Design review of the part built by this model. Coordinates are the model's own, in mm. A direction names the side the tool comes from. Give positions to 0.01 mm unless a question says otherwise; leave off trailing zeros. Loops run counter-clockwise (first coordinate to the right, second up) from the corner with the lowest first, then second, coordinate; pieces in that order, holes last.
from build123d import *

# Parameters (mm, degrees)
F0_W      = 40.2
F0_H      = 40
F1_DEPTH  = 5.5
F2_R      = 2.85
F3_DEPTH  = 3.5
F4_R      = 1.6
F5_DEPTH  = 25
F6_W      = 4.8
F6_H      = 40
F7_DEPTH  = 2
F8_SIZE   = 1.8
F9_R      = 1.6
F10_DEPTH = 25
F11_R     = 2.85
F12_DEPTH = 3.5
F2_W      = 40.2
F2_H      = 40
F13_DEPTH = 6.4
F14_DEPTH = 25
F15_W     = 40.2
F15_H     = 5
F16_DEPTH = 44
F17_R     = 11.1
F17_R_2   = 1.6
F18_DEPTH = 25


with BuildPart() as f1:
    # F0 (on Top) → F1 (new body)
    with BuildSketch(Plane.XY):
        with Locations((20.1, 20)):
            Rectangle(F0_W, F0_H)
    extrude(amount=F1_DEPTH)

    # F2 (on face) → F3 (cut)
    with BuildSketch(Plane.XY.offset(5.5)):
        with Locations((35.2, 6.5)):
            Circle(F2_R)
        with Locations((35.2, 33.5)):
            Circle(F2_R)
        with Locations((5, 33.5)):
            Circle(F2_R)
        with Locations((5, 6.5)):
            Circle(F2_R)
    extrude(amount=-F3_DEPTH, mode=Mode.SUBTRACT)

    # F4 (on face) → F5 (cut)
    with BuildSketch(Plane.XY.offset(5.5)):
        with Locations((35.2, 33.5)):
            Circle(F4_R)
        with Locations((35.2, 6.5)):
            Circle(F4_R)
        with Locations((5, 33.5)):
            Circle(F4_R)
        with Locations((5, 6.5)):
            Circle(F4_R)
    extrude(amount=-F5_DEPTH, mode=Mode.SUBTRACT)

    # F6 (on face) → F7 (join)
    with BuildSketch(Plane(origin=(0, 0, 0), x_dir=(1, 0, 0), z_dir=(0, 0, -1))):
        with Locations((20.1, -20)):
            Rectangle(F6_W, F6_H)
    extrude(amount=F7_DEPTH)

    # F8
    f8_edges = [f1.edges().sort_by_distance(p)[0] for p in [
        (17.7, 20, -2),
        (22.5, 20, -2),
    ]]
    chamfer(f8_edges, length=F8_SIZE)

    # F9 (on face) → F10 (cut)
    with BuildSketch(Plane(origin=(0, 0, -2), x_dir=(1, 0, 0), z_dir=(0, 0, -1))):
        with Locations((20.1, -30)):
            Circle(F9_R)
        with Locations((20.1, -10)):
            Circle(F9_R)
    extrude(amount=-F10_DEPTH, mode=Mode.SUBTRACT)

    # F11 (on face) → F12 (cut)
    with BuildSketch(Plane.XY.offset(5.5)):
        with Locations((20.1, 30)):
            Circle(F11_R)
        with Locations((20.1, 10)):
            Circle(F11_R)
    extrude(amount=-F12_DEPTH, mode=Mode.SUBTRACT)

    # F2 (on face) → F13 (join)
    with BuildSketch(Plane.XY.offset(5.5)):
        with Locations((20.1, 20)):
            Rectangle(F2_W, F2_H)
        with Locations((5, 6.5)):
            Circle(F2_R, mode=Mode.SUBTRACT)
        with Locations((35.2, 6.5)):
            Circle(F2_R, mode=Mode.SUBTRACT)
        with Locations((5, 33.5)):
            Circle(F2_R, mode=Mode.SUBTRACT)
        with Locations((35.2, 33.5)):
            Circle(F2_R, mode=Mode.SUBTRACT)
    extrude(amount=F13_DEPTH)

    # F11 (on face) → F14 (cut)
    with BuildSketch(Plane.XY.offset(5.5)):
        with Locations((20.1, 30)):
            Circle(F11_R)
        with Locations((20.1, 10)):
            Circle(F11_R)
    extrude(amount=F14_DEPTH, mode=Mode.SUBTRACT)

    # F15 (on face) → F16 (join)
    with BuildSketch(Plane.XZ):
        with Locations((20.1, 9.4)):
            Rectangle(F15_W, F15_H)
    extrude(amount=F16_DEPTH)

    # F17 (on face) → F18 (cut)
    with BuildSketch(Plane.XY.offset(11.9)):
        with Locations((20.1, -23)):
            Circle(F17_R)
        with Locations((5.264286, -38.5)):
            Circle(F17_R_2)
        with Locations((34.935714, -38.5)):
            Circle(F17_R_2)
        with Locations((5.264286, -7.5)):
            Circle(F17_R_2)
        with Locations((34.935714, -7.5)):
            Circle(F17_R_2)
    extrude(amount=-F18_DEPTH, mode=Mode.SUBTRACT)


solid = f1.part
Q1. Insertion check: pin 1 (1.7 mm diameter, centred on x = 4.5, y = 32, fed in from +Z); pin 2 (1.7 mm diameter, centred on x = 5, y = 7, fed in from +Z); pin 3 (5 mm diameter, centred on x = 35.2, y = 6.5, fed in from -Z); pin 4 (2.5 mm diameter, centred on x = 20.5, z = 0, fed in from -Y). Each pin has a flat end and moves straight along its axis. Give the tip position at first contact, or say it passes through.
Results:
pin 1: stops at z = 2
pin 2: passes through
pin 3: stops at z = 0
pin 4: stops at y = 0
Q2. Take a section at B-B (y = -38.5). Give the boundary of the cut face in (x, z), plus the area to 3 significant figures.
Results:
outline: (0, 6.9) - (3.66, 6.9) - (3.66, 11.9) - (0, 11.9) - close; (6.86, 6.9) - (33.34, 6.9) - (33.34, 11.9) - (6.86, 11.9) - close; (36.54, 6.9) - (40.2, 6.9) - (40.2, 11.9) - (36.54, 11.9) - close
area: 169 mm2
Q3. Wall thickness on line 1 (Y direction, x = 20.1, z = -1.1); line 2 (Y direction, x = 20.1, z = 7.25); line 3 (X direction, y = 30, z = 5.25): over which ranges is each line inside the solid? List them lowest first.
Results:
line 1: y = 0 to 8.4, 11.6 to 28.4, 31.6 to 40
line 2: y = -44 to -34.1, -11.9 to 7.15, 12.85 to 27.15, 32.85 to 40
line 3: x = 0 to 17.25, 22.95 to 40.2
Q4. Take a section at A-A (z = 11). Give the number of separate pieces and of enclosed holes in the cut face, plus the area to 3 significant figures.
Results:
separate pieces: 1
enclosed holes: 11
area: 2,800 mm2
Q5. Draft analysis for pull direction X (two halves, no side actions). For faces 4 (the face through (0, 8, 7)), 5 (the face through (20, -44, 9)), 6 (the face through (6, 5, 2)), state which applies: pulls with the +X half, pulls with the -X half, needs draft (parallel to the pull), parting line crosses it, or undercut.
Results:
face 4: pulls with the -X half
face 5: needs draft
face 6: undercut
Q6. Tool access review of faces 1 (the face through (6.532, 8.903, 6.881)), 2 (the face through (24, -12, 6.9)), 3 (the face through (40.2, 8, 7)): name each direction out of +Z, -Z, +X, -X, +Y, -Y from which nothing blocks a thin tool from reaching the whole face with its end or side.
Results:
face 1: +Z
face 2: -Z, +X, -X, -Y
face 3: +Z, -Z, +X, +Y, -Y
Q7. Take a section at C-C (y = -23). Give the boundary of the cut face in (x, z).
Results:
outline: (0, 6.9) - (9, 6.9) - (9, 11.9) - (0, 11.9) - close; (31.2, 6.9) - (40.2, 6.9) - (40.2, 11.9) - (31.2, 11.9) - close
Q8. Take a section at D-D (x = 13.5). Give the boundary of the cut face in (y, z), plus the area to 3 significant figures.
Results:
outline: (-44, 6.9) - (-31.92, 6.9) - (-31.92, 11.9) - (-44, 11.9) - close; (-14.08, 6.9) - (0, 6.9) - (0, 0) - (40, 0) - (40, 11.9) - (-14.08, 11.9) - close
area: 607 mm2
